```python
from build123d import *

# Parameters (mm, degrees)
SKETCH1_R                = 19.05
SKETCH1_R_2              = 12.7
BOSS_EXTRUDE1_DEPTH      = 107.95
SKETCH2_R                = 13.97
BOSS_EXTRUDE2_DEPTH      = 6.35
SKETCH8_W                = 19.05
SKETCH8_H                = 82.55
CUT_EXTRUDE6_DEPTH       = 20.05
CUT_EXTRUDE6_DEPTH_BACK  = 20.05
SKETCH7_R                = 6.35
CUT_EXTRUDE4_DEPTH       = 7.35
SKETCH9_W                = 3.175
SKETCH9_H                = 27.952216058
BOSS_EXTRUDE3_DEPTH      = 6.35
BOSS_EXTRUDE3_DEPTH_BACK = 6.35
SKETCH10_R               = 2.38125
CUT_EXTRUDE7_DEPTH       = 29.575


with BuildPart() as part:
    # Sketch1 → Boss-Extrude1 (new body)
    with BuildSketch(Plane(origin=(0, 0, 0), x_dir=(1, 0, 0), z_dir=(0, 1, 0))):
        Circle(SKETCH1_R)
        Circle(SKETCH1_R_2, mode=Mode.SUBTRACT)
    extrude(amount=BOSS_EXTRUDE1_DEPTH)

    # Sketch2 → Boss-Extrude2 (add)
    with BuildSketch(Plane.XZ):
        Circle(SKETCH2_R)
    extrude(amount=-BOSS_EXTRUDE2_DEPTH)

    # Sketch8 → Cut-Extrude6 (cut, two sides)
    with BuildSketch(Plane.XY) as cut_extrude6_sk:
        with Locations((0, 53.975)):
            Rectangle(SKETCH8_W, SKETCH8_H)
    extrude(amount=CUT_EXTRUDE6_DEPTH, mode=Mode.SUBTRACT)
    extrude(cut_extrude6_sk.sketch, amount=-CUT_EXTRUDE6_DEPTH_BACK, mode=Mode.SUBTRACT)

    # Sketch7 → Cut-Extrude4 (cut, through all)
    with BuildSketch(Plane(origin=(0, 6.35, 0), x_dir=(1, 0, 0), z_dir=(0, 1, 0))):
        Circle(SKETCH7_R)
    extrude(amount=-CUT_EXTRUDE4_DEPTH, mode=Mode.SUBTRACT)

    # Sketch9 → Boss-Extrude3 (add, two sides)
    with BuildSketch(Plane(origin=(0, 6.35, 0), x_dir=(1, 0, 0), z_dir=(0, 1, 0))) as boss_extrude3_sk:
        with Locations((-7.9375, -30.473891971)):
            Rectangle(SKETCH9_W, SKETCH9_H)
        with Locations((7.9375, -30.473891971)):
            Rectangle(SKETCH9_W, SKETCH9_H)
        with Locations((7.9375, 30.473891971)):
            Rectangle(SKETCH9_W, SKETCH9_H)
        with Locations((-7.9375, 30.473891971)):
            Rectangle(SKETCH9_W, SKETCH9_H)
    extrude(amount=BOSS_EXTRUDE3_DEPTH)
    extrude(boss_extrude3_sk.sketch, amount=-BOSS_EXTRUDE3_DEPTH_BACK)

    # Sketch10 → Cut-Extrude7 (cut, through all)
    with BuildSketch(Plane.ZY.offset(9.525)):
        with Locations((-38.89375, 6.35)):
            Circle(SKETCH10_R)
        with Locations((38.89375, 6.35)):
            Circle(SKETCH10_R)
    extrude(amount=-CUT_EXTRUDE7_DEPTH, mode=Mode.SUBTRACT)


solid = part.part
```
CAD build for the part. Positions are in the model's coordinates, mm. A direction names the side the tool comes from. Round coordinates to 2 decimals unless told otherwise and drop trailing zeros. Order: outer loops, then holes, each group sorted by start corner. A loop starts at its lowest first (then second) coordinate and runs counter-clockwise, first axis right, second up. Notation, with made-up numbers: (-33.75, 14) - (3.25, 14) arc R21 cw to (3.25, 40) - close; hole circle Ø7 at (13, 65). An arc over 180 degrees is marked (long way). Answer in a Markdown table with one row per item. Add a question column.
(1) Band-saw the part on B-B on z = 21. List the corners of the cut face in (x, y) (3 decimals).
(2) Drop flat-ended pins along their axis: pin 1 Ø5.5 at (y, z) = (6.35, 38.89) entering from -X (3 decimals); pin 2 Ø1.5 at (x, z) = (12, 1.5) entering from -Y; pin 3 Ø6.5 at (y, z) = (51, 10.5) entering from +X; pin 4 Ø7.5 at (x, z) = (5.5, 6) entering from +Y. Give the stop position or say it passes through.
(3) Band-saw the part on D-D on z = 0. List the corners of the cut face in (x, y), and give its area (3 significant figures).
(4) Band-saw the part on C-C on x = 0. List the corners of the cut face in (y, z).
(5) Probe L1, parallel to Z at x = 8, y = 6; L2, parallel to X at y = 5.25, z = 0; L3, parallel to Y at x = -7.5, z = 17. List the from-to ranges inside material, lowest first. Write a range as [from, to].
(6) Mould opens along Z. For faces 1 (the face through (8, 6, -44.45)), 2 (the face through (-6.5, 12.7, 22.2)), 3 (the face through (-7.96, 4.237, 39.993)) say: +Z half, -Z half, draft (parallel to the pull), parting line (faces both ways), or undercut.
(7) Band-saw the part on A-A on y = 72. List the corners of the cut face in (x, z) (3 decimals), and give its area (3 significant figures).
(8) 3-axis set-ups, long thin cutter, end or side, ignore diameter. For faces 4 (the face through (9.525, 6, -30)), 5 (the face through (-6.35, 6, 31)), 6 (the face through (-9.525, 53, 12)): which of +Z, -Z, +X, -X, +Y, -Y reach the whole face in a straight line?
Data:
| question | item | result |
|---|---|---|
| 1 | outline | (-9.525, 0) - (-6.35, 0) - (-6.35, 12.7) - (-9.525, 12.7) - close; (6.35, 0) - (9.525, 0) - (9.525, 12.7) - (6.35, 12.7) - close |
| 2 | pin 1 | stops at x = -9.525 |
| 2 | pin 2 | stops at y = 0 |
| 2 | pin 3 | stops at x = 17.62 |
| 2 | pin 4 | stops at y = 6.35 |
| 3 | outline | (-19.05, 0) - (-6.35, 0) - (-6.35, 6.35) - (-12.7, 6.35) - (-12.7, 107.95) - (-19.05, 107.95) - close; (6.35, 0) - (19.05, 0) - (19.05, 107.95) - (12.7, 107.95) - (12.7, 6.35) - (6.35, 6.35) - close |
| 3 | area | 1,450 mm^2 |
| 4 | outline | (0, -19.05) - (12.7, -19.05) - (12.7, -12.7) - (6.35, -12.7) - (6.35, -6.35) - (0, -6.35) - close; (0, 6.35) - (6.35, 6.35) - (6.35, 12.7) - (12.7, 12.7) - (12.7, 19.05) - (0, 19.05) - close; (95.25, -19.05) - (107.95, -19.05) - (107.95, -12.7) - (95.25, -12.7) - close; (95.25, 12.7) - (107.95, 12.7) - (107.95, 19.05) - (95.25, 19.05) - close |
| 5 | L1 | z = [-44.45, -41.25], [-36.54, 36.54], [41.25, 44.45] |
| 5 | L2 | x = [-19.05, -6.35], [6.35, 19.05] |
| 5 | L3 | y = [0, 12.7], [95.25, 107.95] |
| 6 | face 1 | -Z half |
| 6 | face 2 | draft |
| 6 | face 3 | undercut |
| 7 | outline | (-9.525, -16.498) - (-9.525, -8.4) arc R12.7 cw to (-9.525, 8.4) - (-9.525, 16.498) arc R19.05 ccw to start; (9.525, -16.498) arc R19.05 ccw to (9.525, 16.498) - (9.525, 8.4) arc R12.7 cw to (9.525, -8.4) - close |
| 7 | area | 373 mm^2 |
| 8 | face 4 | -Z, +X, +Y, -Y |
| 8 | face 5 | +Z, +Y, -Y |
| 8 | face 6 | +Z, -Z |
